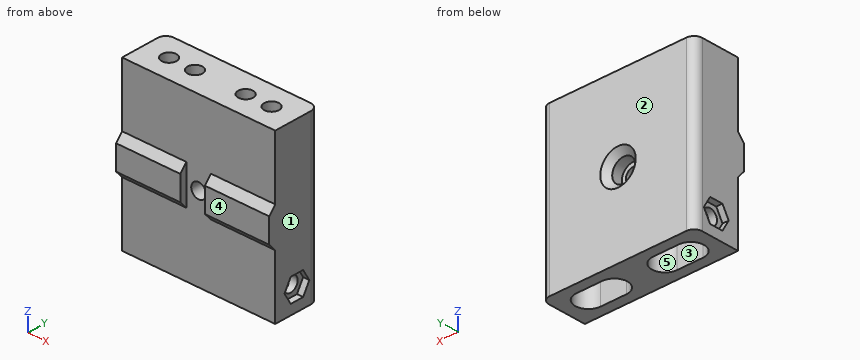
```python
from build123d import *

# Parameters (mm, degrees)
SKETCH_W        = 37.2
SKETCH_H        = 11.3
PAD_DEPTH       = 40
SKETCH001_R     = 1.8
PAD001_DEPTH    = 2.5
PAD002_DEPTH    = 37.2
SKETCH003_R     = 1.8
POCKET_DEPTH    = 12.861
SKETCH004_W     = 6
SKETCH004_H     = 9.48
POCKET001_DEPTH = 1.56
SKETCH005_R     = 2.8
POCKET002_DEPTH = 4
SKETCH006_R     = 1.8
POCKET003_DEPTH = 37.201
POCKET004_DEPTH = 1.5
POCKET005_DEPTH = 1.5
FILLET_R        = 2
CHAMFER_SIZE    = 1.5


with BuildPart() as part:
    # Sketch → Pad (new body)
    with BuildSketch(Plane.XY):
        Rectangle(SKETCH_W, SKETCH_H)
        with BuildLine():
            ThreePointArc((-12.45, 3.15), (-15.6, 0), (-12.45, -3.15))
            Line((-12.45, -3.15), (-6.15, -3.15))
            ThreePointArc((-6.15, -3.15), (-3, 0), (-6.15, 3.15))
            Line((-6.15, 3.15), (-12.45, 3.15))
        make_face(mode=Mode.SUBTRACT)
        with BuildLine():
            ThreePointArc((12.45, -3.15), (15.6, 0), (12.45, 3.15))
            Line((12.45, 3.15), (6.15, 3.15))
            ThreePointArc((6.15, 3.15), (3, 0), (6.15, -3.15))
            Line((6.15, -3.15), (12.45, -3.15))
        make_face(mode=Mode.SUBTRACT)
    extrude(amount=PAD_DEPTH)

    # Sketch001 (on Face14 of Pad) → Pad001 (join)
    with BuildSketch(Plane.XY.offset(40)):
        with BuildLine():
            ThreePointArc((-12.45, 3.15), (-15.6, 0), (-12.45, -3.15))
            Line((-12.45, -3.15), (-6.15, -3.15))
            ThreePointArc((-6.15, -3.15), (-3, 0), (-6.15, 3.15))
            Line((-6.15, 3.15), (-12.45, 3.15))
        make_face()
        with Locations((-12.45, 0)):
            Circle(SKETCH001_R, mode=Mode.SUBTRACT)
        with Locations((-6.15, 0)):
            Circle(SKETCH001_R, mode=Mode.SUBTRACT)
        with BuildLine():
            ThreePointArc((12.45, -3.15), (15.6, 0), (12.45, 3.15))
            Line((12.45, 3.15), (6.15, 3.15))
            ThreePointArc((6.15, 3.15), (3, 0), (6.15, -3.15))
            Line((6.15, -3.15), (12.45, -3.15))
        make_face()
        with Locations((6.15, 0)):
            Circle(SKETCH001_R, mode=Mode.SUBTRACT)
        with Locations((12.45, 0)):
            Circle(SKETCH001_R, mode=Mode.SUBTRACT)
    extrude(amount=-PAD001_DEPTH)

    # Sketch002 (on Face3 of Pad001) → Pad002 (join)
    with BuildSketch(Plane.YZ.offset(18.6)):
        Polygon((-5.65, 24.74), (-5.65, 15.26), (-7.21, 17.06), (-7.21, 22.94), align=None)
    extrude(amount=-PAD002_DEPTH)

    # Sketch003 (on Face22 of Pad002) → Pocket (cut, through all)
    with BuildSketch(Plane.XZ.offset(7.21)):
        with Locations((0, 20)):
            Circle(SKETCH003_R)
    extrude(amount=-POCKET_DEPTH, mode=Mode.SUBTRACT)

    # Sketch004 (on Face21 of Pocket) → Pocket001 (cut)
    with BuildSketch(Plane.XZ.offset(7.21)):
        with Locations((0, 20)):
            Rectangle(SKETCH004_W, SKETCH004_H)
    extrude(amount=-POCKET001_DEPTH, mode=Mode.SUBTRACT)

    # Sketch005 (on Face1 of Pocket001) → Pocket002 (cut)
    with BuildSketch(Plane(origin=(0, 5.65, 0), x_dir=(-1, 0, 0), z_dir=(0, 1, 0))):
        with Locations((0, 20)):
            Circle(SKETCH005_R)
    extrude(amount=-POCKET002_DEPTH, mode=Mode.SUBTRACT)

    # Sketch006 (on Face5 of Pocket002) → Pocket003 (cut, through all)
    with BuildSketch(Plane.YZ.offset(18.6)):
        with Locations((0, 5.2)):
            Circle(SKETCH006_R)
    extrude(amount=-POCKET003_DEPTH, mode=Mode.SUBTRACT)

    # Sketch007 (on Face5 of Pocket003) → Pocket004 (cut)
    with BuildSketch(Plane.YZ.offset(18.6)):
        Polygon((1.616581, 8), (-1.616581, 8), (-3.233162, 5.2), (-1.616581, 2.4), (1.616581, 2.4), (3.233162, 5.2), align=None)
    extrude(amount=-POCKET004_DEPTH, mode=Mode.SUBTRACT)

    # Sketch008 (on Face2 of Pocket004) → Pocket005 (cut)
    with BuildSketch(Plane(origin=(-18.6, 0, 0), x_dir=(0, -1, 0), z_dir=(-1, 0, 0))):
        Polygon((1.616581, 8), (-1.616581, 8), (-3.233162, 5.2), (-1.616581, 2.4), (1.616581, 2.4), (3.233162, 5.2), align=None)
    extrude(amount=-POCKET005_DEPTH, mode=Mode.SUBTRACT)

    # Fillet
    fillet_edges = [part.edges().sort_by_distance(p)[0] for p in [
        (-18.6, 5.65, 20),
        (18.6, 5.65, 20),
    ]]
    fillet(fillet_edges, radius=FILLET_R)

    # Chamfer
    chamfer_edges = [part.edges().sort_by_distance(p)[0] for p in [
        (2.8, 5.65, 20),
    ]]
    chamfer(chamfer_edges, length=CHAMFER_SIZE)


solid = part.part
```
Can you work these out from the model? Positions are in its coordinate system, mm. Face numbers are marked on the shaded views. A direction names the side the tool comes from. Round coordinates to 2 decimals unless told otherwise and drop trailing zeros. Loops run counter-clockwise (first coordinate to the right, second up) from the corner with the lowest first, then second, coordinate; pieces in that order, holes last. Notation, with made-up numbers: M 40.5,67.25 L 84.5,67.25 A5 ccw 84.5,74.25 Z; hole C -13.5,80 d6. An arc over 180 degrees is marked long. Write item = value, one per line. Start each with the question number.
(1) Which directions (+Z, -Z, +X, -X, +Y, -Y) give clear straight access to the entire face, cutting with the end or side of a thin tool? Please do the marked faces 4 and 5.
(2) If we mould it in two halves opening along Y, with no side actions, what happens to the marked faces 1, 2 and 3? For each: released by +Y, released by -Y, zero draft, split by the parting line, or undercut.
(3) I'm going to push flat-ended pins straight in: P1, Ø7, axis at x = -11, y = 1, coming from the -Z side; P2, Ø4.5, axis at x = 0, z = 20, coming from the +Y side; P3, Ø4, axis at x = 0, z = 20, coming from the -Y side; P4, Ø6, axis at x = -12.45, y = 0, coming from the -Z side. Where does each tip first touch, or does it pass through?
(4) I need wall thicknesses on line 1 along Z through (x, y) = (15.8, 0); line 2 along Y through (x, z) = (12.5, 30); line 3 along Z through (x, y) = (0, -4). Which ranges of each line are inside material? Lowest first, please.
(5) Suppose I cut it at B-B on z = 33. Write out the boundary of the cut face in (x, y).
(6) Suppose I cut it at D-D on y = 0. Give the number of separate pieces and of enclosed holes in the cut face, plus the area to 3 significant figures.
(7) Suppose I cut it at A-A on x = 0. Write out the boundary of the cut face in (y, z).
Answer block:
q1.face_4 = +Z, -Z, +X, -X, -Y
q1.face_5 = -Z
q2.face_1 = zero draft
q2.face_2 = released by +Y
q2.face_3 = undercut
q3.P1 = 0
q3.P2 = 1.65
q3.P3 = -5.65
q3.P4 = 37.5
q4.line_1 = 0 to 3.4, 7 to 40
q4.line_2 = -5.65 to -3.15, 3.15 to 5.65
q4.line_3 = 0 to 18.2, 21.8 to 40
q5.outline = M -18.6,-5.65 L 18.6,-5.65 L 18.6,3.65 A2 ccw 16.6,5.65 L -16.6,5.65 A2 ccw -18.6,3.65 Z; hole M -12.45,-3.15 L -6.15,-3.15 A3.15 ccw -6.15,3.15 L -12.45,3.15 A3.15 ccw Z; hole M 6.15,-3.15 L 12.45,-3.15 A3.15 ccw 12.45,3.15 L 6.15,3.15 A3.15 ccw Z
q6.separate_pieces = 8
q6.enclosed_holes = 1
q6.area = 448 mm²
q7.outline = M -5.65,0 L 5.65,0 L 5.65,15.7 L 4.15,17.2 L 1.65,17.2 L 1.65,18.2 L -5.65,18.2 Z; M -5.65,21.8 L 1.65,21.8 L 1.65,22.8 L 4.15,22.8 L 5.65,24.3 L 5.65,40 L -5.65,40 Z; hole C 0,5.2 d3.6
